Here's how the part is built. I have some questions about the finished solid (model axes, mm). A direction names the side the tool comes from. Round coordinates to 2 decimals unless told otherwise and drop trailing zeros. Order: outer loops, then holes, each group sorted by start corner. A loop starts at its lowest first (then second) coordinate and runs counter-clockwise, first axis right, second up. Notation, with made-up numbers: (50.5, 83) - (74.5, 83) arc R20 ccw to (74.5, 119) - close; hole circle Ø1 at (-22, 54). An arc over 180 degrees is marked (long way). Answer as a JSON object with one key per item and string values.
```python
from build123d import *

# Parameters (mm, degrees)
SKETCH1_W           = 71.12
SKETCH1_H           = 59.69
BOSS_EXTRUDE1_DEPTH = 2
SKETCH2_R           = 2
CUT_EXTRUDE1_DEPTH  = 2
SKETCH3_W           = 14
SKETCH3_H           = 10
BOSS_EXTRUDE2_DEPTH = 5
SKETCH4_W           = 10
SKETCH4_H           = 10
BOSS_EXTRUDE3_DEPTH = 13
CUT_EXTRUDE2_DEPTH  = 49.882651319
SKETCH8_W           = 13
SKETCH8_H           = 4
CUT_EXTRUDE3_DEPTH  = 7
CHAMFER1_SIZE       = 3
SKETCH9_W           = 4.4
SKETCH9_H           = 3.6
CUT_EXTRUDE4_DEPTH  = 8
SKETCH10_R          = 2
CUT_EXTRUDE5_DEPTH  = 1


with BuildPart() as part:
    # Sketch1 → Boss-Extrude1 (new body)
    with BuildSketch(Plane(origin=(0, 0, 0), x_dir=(1, 0, 0), z_dir=(0, 1, 0))):
        Rectangle(SKETCH1_W, SKETCH1_H)
    extrude(amount=BOSS_EXTRUDE1_DEPTH)

    # Sketch2 → Cut-Extrude1 (cut)
    with BuildSketch(Plane(origin=(0, 2, 0), x_dir=(1, 0, 0), z_dir=(0, 1, 0))):
        with Locations(Location((-30.48, 24.765, 0), (0, 0, 270))):
            Circle(SKETCH2_R)
        with Locations(Location((30.48, 24.765, 0), (0, 0, 270))):
            Circle(SKETCH2_R)
        with Locations(Location((30.48, -24.765, 0), (0, 0, 270))):
            Circle(SKETCH2_R)
        with Locations(Location((-30.48, -24.765, 0), (0, 0, 270))):
            Circle(SKETCH2_R)
    extrude(amount=-CUT_EXTRUDE1_DEPTH, mode=Mode.SUBTRACT)

    # Sketch3 → Boss-Extrude2 (add)
    with BuildSketch(Plane(origin=(0, 2, 0), x_dir=(1, 0, 0), z_dir=(0, 1, 0))):
        with Locations((-18.56, -23.845)):
            Rectangle(SKETCH3_W, SKETCH3_H)
        with Locations((18.56, -23.845)):
            Rectangle(SKETCH3_W, SKETCH3_H)
    extrude(amount=BOSS_EXTRUDE2_DEPTH)

    # Sketch4 → Boss-Extrude3 (add)
    with BuildSketch(Plane(origin=(0, 2, 0), x_dir=(1, 0, 0), z_dir=(0, 1, 0))):
        with Locations((29.56, 4.845)):
            Rectangle(SKETCH4_W, SKETCH4_H)
    extrude(amount=BOSS_EXTRUDE3_DEPTH)

    # Sketch7 → Cut-Extrude2 (cut, through all)
    with BuildSketch(Plane.XY.offset(0.155)):
        Polygon((26.56, 15), (24.56, 6), (24.56, 15), align=None)
        Polygon((34.56, 6), (32.56, 15), (34.56, 15), align=None)
    extrude(amount=-CUT_EXTRUDE2_DEPTH, mode=Mode.SUBTRACT)

    # Sketch8 → Cut-Extrude3 (cut)
    with BuildSketch(Plane.XY.offset(28.845)):
        with Locations((-18.56, 4.5)):
            Rectangle(SKETCH8_W, SKETCH8_H)
        with Locations((18.56, 4.5)):
            Rectangle(SKETCH8_W, SKETCH8_H)
    extrude(amount=-CUT_EXTRUDE3_DEPTH, mode=Mode.SUBTRACT)

    # Chamfer1
    chamfer1_edges = [part.edges().sort_by_distance(p)[0] for p in [
        (-18.56, 7, 18.845),
        (18.56, 7, 18.845),
    ]]
    chamfer(chamfer1_edges, length=CHAMFER1_SIZE)

    # Sketch9 → Cut-Extrude4 (cut)
    with BuildSketch(Plane(origin=(34.56, 0, 0), x_dir=(0, 0, -1), z_dir=(1, 0, 0))):
        with Locations((7.345, 4)):
            Rectangle(SKETCH9_W, SKETCH9_H)
        with Locations((2.345, 4)):
            Rectangle(SKETCH9_W, SKETCH9_H)
    extrude(amount=-CUT_EXTRUDE4_DEPTH, mode=Mode.SUBTRACT)

    # Sketch10 → Cut-Extrude5 (cut)
    with BuildSketch(Plane(origin=(0, 15, 0), x_dir=(1, 0, 0), z_dir=(0, 1, 0))):
        with Locations(Location((29.56, 7.345, 0), (0, 0, 270))):
            Circle(SKETCH10_R)
        with Locations(Location((29.56, 2.345, 0), (0, 0, 90))):
            Circle(SKETCH10_R)
    extrude(amount=-CUT_EXTRUDE5_DEPTH, mode=Mode.SUBTRACT)


solid = part.part
```
1. Imagine slicing it at D-D (x = -19). List the corners of the cut face in (y, z) for me (3 decimals).
Responses:
{"outline": "(0, -29.845) - (2, -29.845) - (2, 18.845) - (4, 18.845) - (7, 21.845) - (7, 28.845) - (6.5, 28.845) - (6.5, 21.845) - (2.5, 21.845) - (2.5, 28.845) - (2, 28.845) - (2, 29.845) - (0, 29.845) - close"}
2. Thinking about a two-plate mould opening in X: for faces 1 (the face through (31.543, 14.507, -7.605)), 2 (the face through (-11.56, 4, 24)), 3 (the face through (34.56, 4, -4.8)), 4 (the face through (31, 4, -5.145)), which applies, pulls with the +X half, pulls with the -X half, needs draft (parallel to the pull), parting line crosses it, or undercut?
Responses:
{"face 1": "undercut", "face 2": "undercut", "face 3": "pulls with the +X half", "face 4": "needs draft"}
3. If I drill on L1, parallel to Z at x = 31.5, y = 5.75 (3 decimals); L2, parallel to X at y = 1.75, z = -25; L3, parallel to Y at x = 10, z = 18.5, over which ranges is the centre line in solid material (lowest first)? Write a range as [from, to].
Responses:
{"L1": "[-9.845, -9.545], [-5.145, -4.545], [-0.145, 0.155]", "L2": "[-35.56, -32.47], [-28.49, 28.49], [32.47, 35.56]", "L3": "[0, 2]"}
4. Imagine slicing it at B-B (z = 26). List the corners of the cut face in (x, y) for me, plus the area to 3 significant figures.
Responses:
{"outline": "(-35.56, 0) - (-32.05, 0) - (-32.05, 2) - (-35.56, 2) - close; (-28.91, 0) - (28.91, 0) - (28.91, 2) - (25.56, 2) - (25.56, 7) - (11.56, 7) - (11.56, 2) - (-11.56, 2) - (-11.56, 7) - (-25.56, 7) - (-25.56, 2) - (-28.91, 2) - close; (32.05, 0) - (35.56, 0) - (35.56, 2) - (32.05, 2) - close; hole (-25.06, 2.5) - (-12.06, 2.5) - (-12.06, 6.5) - (-25.06, 6.5) - close; hole (12.06, 2.5) - (25.06, 2.5) - (25.06, 6.5) - (12.06, 6.5) - close", "area": "166 mm2"}
5. Imagine slicing it at A-A (x = -30.48). List the corners of the cut face in (y, z) for me (3 decimals), plus the area to 3 significant figures.
Responses:
{"outline": "(0, -29.845) - (2, -29.845) - (2, -26.765) - (0, -26.765) - close; (0, -22.765) - (2, -22.765) - (2, 22.765) - (0, 22.765) - close; (0, 26.765) - (2, 26.765) - (2, 29.845) - (0, 29.845) - close", "area": "103 mm2"}
6. For faces 5 (the face through (-25.56, 4, 24)), 6 (the face through (11.56, 4, 24)), 7 (the face through (12.06, 4, 25)), 8 (the face through (31, 4, -9.545)), which set-ups out of +Z, -Z, +X, -X, +Y, -Y let a thin tool reach every point of the face, with its end or its side?
Responses:
{"face 5": "+Z, -Z, -X, +Y", "face 6": "+Z, -Z, +Y", "face 7": "+Z", "face 8": "+X"}
7. For P1, Ø3, axis at x = 19.5, z = -6.5, coming from the +Y side; P2, Ø2, axis at y = 3.5, z = -2.5, coming from the -X side; P3, Ø1.2, axis at y = 3.5, z = -4.5, coming from the +X side; P4, Ø2.5, axis at x = -30.48, z = -24.765, coming from the -Y side, each with a flat end and sliding along its axis, tell me the tip position at first contact or that it passes through.
Responses:
{"P1": "y = 2", "P2": "x = 24.56", "P3": "x = 34.56", "P4": "through"}
8. Imagine slicing it at C-C (x = 29.56). Give the number of separate pieces and of enclosed holes in the cut face, plus the area to 3 significant figures.
Responses:
{"separate pieces": "3", "enclosed holes": "2", "area": "195 mm2"}
